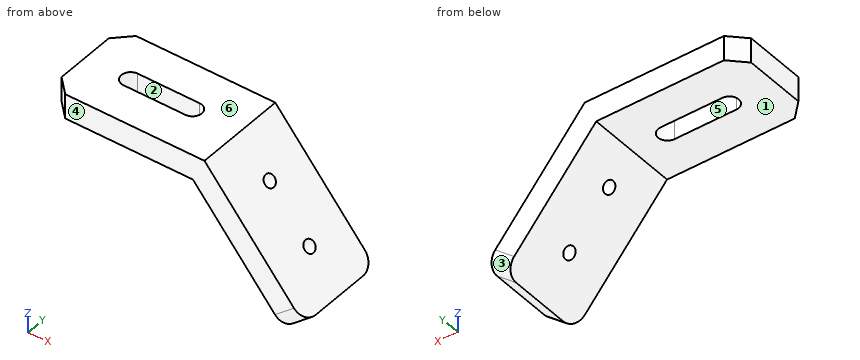
from build123d import *

# Parameters (mm, degrees)
F1_DEPTH = 15
F3_DEPTH = 43.4455230334
F5_D     = 4
F6_R     = 5
F7_SIZE  = 5


with BuildPart() as f1:
    # F0 (on Front) → F1 (new body, symmetric)
    with BuildSketch(Plane.XZ):
        Polygon((0, 8), (0, 0), (46.2695387348, 0), (76.0110249394, -35.4445230334), (82.1393804843, -30.3022221559), (50, 8), align=None)
    extrude(amount=F1_DEPTH, both=True)

    # F2 (on face) → F3 (cut, through all)
    with BuildSketch(Plane.XY.offset(8)):
        with BuildLine():
            ThreePointArc((14.6969384567, 3), (11.6969384567, 0), (14.6969384567, -3))
            Line((14.6969384567, -3), (34.6969384567, -3))
            ThreePointArc((34.6969384567, -3), (37.6969384567, 0), (34.6969384567, 3))
            Line((34.6969384567, 3), (14.6969384567, 3))
        make_face()
    extrude(amount=-F3_DEPTH, mode=Mode.SUBTRACT)

    # F5 (through all)
    with Locations(Plane(origin=(33.2804354537, 0, 27.9256011146), x_dir=(0, 1, 0), z_dir=(0.7660444431, 0, 0.6427876097))):
        with Locations((0, -41.0110249394), (0, -61.0110249394)):
            Hole(F5_D / 2)

    # F6
    f6_edges = [f1.edges().sort_by_distance(p)[0] for p in [
        (79.075203, -15, -32.873373),
        (79.075203, 15, -32.873373),
    ]]
    fillet(f6_edges, radius=F6_R)

    # F7
    f7_edges = [f1.edges().sort_by_distance(p)[0] for p in [
        (0, -15, 4),
        (0, 15, 4),
    ]]
    chamfer(f7_edges, length=F7_SIZE)


solid = f1.part
Can you work these out from the model? Positions are in its coordinate system, mm. Face numbers are marked on the shaded views. A direction names the side the tool comes from. Give positions to 0.01 mm unless a question says otherwise; leave off trailing zeros. Write each loop counter-clockwise with the first axis right and the second up, starting at its lowest first coordinate (ties: lowest second). Pieces come first, ordered by that corner, then holes. Notation, with made-up numbers: M 36,67 L 47,67 A10 ccw 47,78 Z; hole C 62.5,4.5 d2. An arc over 180 degrees is marked long. Answer in a Markdown table with one row per item. Add a question column.
Item 1: On a 3-axis mill with a long thin cutter (end or side, diameter ignored), from which of +Z, -Z, +X, -X, +Y, -Y can I reach the whole of each face in a straight line? I mean the marked faces 1, 2 and 3. Say none if no direction works.
Item 2: We'd pull the mould along Y, two halves only. Please class the marked faces 4, 5 and 6: released by +Y, released by -Y, zero draft, split by the parting line, or undercut.
Item 3: Imagine slicing it at C-C, the plane y = 6.5. Write out the boundary of the cut face in (x, z).
Item 4: Please list where these lines run through material, in increasing order: L1, parallel to Z at x = 6, y = -6.5; L2, parallel to Y at x = 69, z = -23; L3, parallel to X at y = 12, z = -1.
Item 5: For pin 1 Ø1 at (x, y) = (48.5, 9) entering from -Z; pin 2 Ø2 at (y, z) = (0, -9) entering from -X; pin 3 Ø6 at (y, z) = (1.5, -6.5) entering from +X, each with a flat end and sliding along its axis, tell me the tip position at first contact or that it passes through.
Item 6: Imagine slicing it at D-D, the plane z = -1. Write out the boundary of the cut face in (x, y), plus the area to 3 significant figures.
Item 7: Imagine slicing it at B-B, the plane x = 35.5. Write out the boundary of the cut face in (y, z).
Item 8: Imagine slicing it at A-A, the plane y = 0. Write out the boundary of the cut face in (x, z).
Evaluation:
| question | item | result |
|---|---|---|
| 1 | face 1 | -Z, -X, +Y, -Y |
| 1 | face 2 | +Z, -Z |
| 1 | face 3 | -Z, +X, +Y |
| 2 | face 4 | released by -Y |
| 2 | face 5 | undercut |
| 2 | face 6 | zero draft |
| 3 | outline | M 0,0 L 46.27,0 L 76.01,-35.44 L 82.14,-30.3 L 50,8 L 0,8 Z |
| 4 | L1 | z = 0 to 8 |
| 4 | L2 | y = -15 to -1.75, 1.75 to 15 |
| 4 | L3 | x = 47.11 to 57.55 |
| 5 | pin 1 | stops at z = -3.25 |
| 5 | pin 2 | stops at x = 55 |
| 5 | pin 3 | stops at x = 64.68 |
| 6 | outline | M 47.11,-15 L 57.55,-15 L 57.55,15 L 47.11,15 Z |
| 6 | area | 313 mm² |
| 7 | outline | M -15,0 L -2.89,0 L -2.89,8 L -15,8 Z; M 2.89,0 L 15,0 L 15,8 L 2.89,8 Z |
| 8 | outline | M 0,0 L 11.7,0 L 11.7,8 L 0,8 Z; M 37.7,0 L 46.27,0 L 52.23,-7.1 L 58.36,-1.96 L 50,8 L 37.7,8 Z; M 54.8,-10.17 L 65.08,-22.42 L 71.21,-17.28 L 60.93,-5.02 Z; M 67.65,-25.49 L 76.01,-35.44 L 82.14,-30.3 L 73.78,-20.34 Z |
